from build123d import *

# Parameters (mm, degrees)
F1_DEPTH = 3
F2_DEPTH = 34
F4_DEPTH = 3


with BuildPart() as f1:
    # F0 (on Top) → F1 (new body)
    with BuildSketch(Plane.XY):
        with BuildLine():
            Line((15.75, -23.5), (15.75, 0))
            ThreePointArc((15.75, 0), (0, 15.75), (-15.75, 0))
            Line((-15.75, 0), (-15.75, -23.5))
            ThreePointArc((-15.75, -23.5), (0, -39.25), (15.75, -23.5))
        make_face()
        with BuildLine():
            ThreePointArc((-12.75, 0), (0, 12.75), (12.75, 0))
            Line((12.75, 0), (12.75, -23.5))
            ThreePointArc((12.75, -23.5), (0, -36.25), (-12.75, -23.5))
            Line((-12.75, -23.5), (-12.75, 0))
        make_face(mode=Mode.SUBTRACT)
        with BuildLine():
            ThreePointArc((-12.75, 0), (0, -12.75), (12.75, 0))
            ThreePointArc((12.75, 0), (0, 12.75), (-12.75, 0))
        make_face()
        with BuildLine():
            Line((12.75, -23.5), (12.75, 0))
            ThreePointArc((12.75, 0), (0, -12.75), (-12.75, 0))
            Line((-12.75, 0), (-12.75, -23.5))
            ThreePointArc((-12.75, -23.5), (0, -36.25), (12.75, -23.5))
        make_face()
    extrude(amount=F1_DEPTH)

    # F0 (on Top) → F2 (join)
    with BuildSketch(Plane.XY):
        with BuildLine():
            Line((15.75, -23.5), (15.75, 0))
            ThreePointArc((15.75, 0), (0, 15.75), (-15.75, 0))
            Line((-15.75, 0), (-15.75, -23.5))
            ThreePointArc((-15.75, -23.5), (0, -39.25), (15.75, -23.5))
        make_face()
        with BuildLine():
            ThreePointArc((-12.75, 0), (0, 12.75), (12.75, 0))
            Line((12.75, 0), (12.75, -23.5))
            ThreePointArc((12.75, -23.5), (0, -36.25), (-12.75, -23.5))
            Line((-12.75, -23.5), (-12.75, 0))
        make_face(mode=Mode.SUBTRACT)
    extrude(amount=-F2_DEPTH)

    # F3 (on face) → F4 (join)
    with BuildSketch(Plane(origin=(0, 0, -34), x_dir=(1, 0, 0), z_dir=(0, 0, -1))):
        with BuildLine():
            ThreePointArc((-15.75, 0), (0, -15.75), (15.75, 0))
            Line((15.75, 0), (15.75, 23.5))
            ThreePointArc((15.75, 23.5), (0, 39.25), (-15.75, 23.5))
            Line((-15.75, 23.5), (-15.75, 0))
        make_face()
        with BuildLine():
            Line((-14.35, 0), (-14.35, 23.5))
            ThreePointArc((-14.35, 23.5), (0, 37.85), (14.35, 23.5))
            Line((14.35, 23.5), (14.35, 0))
            ThreePointArc((14.35, 0), (0, -14.35), (-14.35, 0))
        make_face(mode=Mode.SUBTRACT)
    extrude(amount=F4_DEPTH)


solid = f1.part
Work out the finished part from the listing and answer in its coordinate system (mm). A direction names the side the tool comes from. Give positions to 0.01 mm unless a question says otherwise; leave off trailing zeros. Loops run counter-clockwise (first coordinate to the right, second up) from the corner with the lowest first, then second, coordinate; pieces in that order, holes last. Notation, with made-up numbers: (87, 17.5) -> (92, 17.5) arc R28 ccw to (92, 43.5) -> close; hole circle Ø6 at (2.5, 73.25). An arc over 180 degrees is marked (long way). Use a Markdown table: item, result. Add a question column.
1) The part is cut by section A-A, the plane z = -10.5. Determine the outline of the cut face in (x, y).
2) The part is cut by section B-B, the plane y = -6.5. Determine the outline of the cut face in (x, z), plus the area to 3 significant figures.
3) The part is cut by section C-C, the plane x = 0. Determine the outline of the cut face in (y, z).
4) For a pull along Y with two mould halves and no side action, classify faces 3 (the cylindrical face through (-0.346, 15.746, -16.72)), 4 (the flat face through (14.35, -12, -35)), 5 (the flat face through (-13, -12, -34)), 6 (the flat face through (15, -12, -37)) as +Y half, -Y half, draft (parallel to the pull), parting line (faces both ways), or undercut.
5) Consider line 1 along X through (y, z) = (-5.5, -1.5); line 2 along Y through (x, z) = (0.5, -2); line 3 along Z through (x, y) = (-7, -19). Determine where each line is inside the solid, lowest interval first.
6) Which of the six approach directions +Z, -Z, +X, -X, +Y, -Y give full straight-line access (tool end or side, diameter ignored) to faces 1 (the flat face through (15.75, -12, -17)), 2 (the cylindrical face through (0.28, -36.247, -16.762))?
7) Each of these flat-tipped pins is pushed along its axis until it touches: P1, Ø6, axis at x = -5, z = -20, coming from the -Y side; P2, Ø1.5, axis at x = 11.5, y = 3, coming from the -Z side; P3, Ø14.5, axis at x = 6, y = -20, coming from the -Z side. Where does it stop, or does it pass through?
Reported:
| question | item | result |
|---|---|---|
| 1 | outline | (-15.75, -23.5) arc R15.75 ccw to (15.75, -23.5) -> (15.75, 0) arc R15.75 ccw to (-15.75, 0) -> close; hole (-12.75, -23.5) arc R12.75 ccw to (12.75, -23.5) -> (12.75, 0) arc R12.75 ccw to (-12.75, 0) -> close |
| 2 | outline | (-15.75, -37) -> (-14.35, -37) -> (-14.35, -34) -> (-12.75, -34) -> (-12.75, 0) -> (12.75, 0) -> (12.75, -34) -> (14.35, -34) -> (14.35, -37) -> (15.75, -37) -> (15.75, 3) -> (-15.75, 3) -> close |
| 2 | area | 307 mm^2 |
| 3 | outline | (-39.25, -37) -> (-37.85, -37) -> (-37.85, -34) -> (-36.25, -34) -> (-36.25, 0) -> (12.75, 0) -> (12.75, -34) -> (14.35, -34) -> (14.35, -37) -> (15.75, -37) -> (15.75, 3) -> (-39.25, 3) -> close |
| 4 | face 3 | +Y half |
| 4 | face 4 | undercut |
| 4 | face 5 | undercut |
| 4 | face 6 | draft |
| 5 | line 1 | x = -15.75 to -12.75, 12.75 to 15.75 |
| 5 | line 2 | y = -39.24 to -36.24, 12.74 to 15.74 |
| 5 | line 3 | z = 0 to 3 |
| 6 | face 1 | +Z, -Z, +X, +Y, -Y |
| 6 | face 2 | -Z |
| 7 | P1 | stops at y = -39.12 |
| 7 | P2 | stops at z = 0 |
| 7 | P3 | stops at z = -34 |
